Build history of the part. All positions in model axes, mm. A direction names the side the tool comes from. Round coordinates to 2 decimals unless told otherwise and drop trailing zeros. Write each loop counter-clockwise with the first axis right and the second up, starting at its lowest first coordinate (ties: lowest second). Pieces come first, ordered by that corner, then holes. Notation, with made-up numbers: (26, -35) -> (54, -35) arc R22 ccw to (54, -28) -> close; hole circle Ø2 at (86.5, 53). An arc over 180 degrees is marked (long way). Return JSON: item names as keys, results as strings.
from build123d import *

# Parameters (mm, degrees)
SKETCH_1_R          = 20
EXTRUDE_1_DEPTH     = 30
EXTRUDE_2_DEPTH     = 10
EXTRUDE_START       = -10
EXTRUDE_3_DEPTH     = 10
CUT_EXTRUDE_1_DEPTH = 30
SKETCH_6_W          = 120
SKETCH_6_H          = 10
CUT_EXTRUDE_2_DEPTH = 20
SKETCH_7_R          = 20
EXTRUDE_4_DEPTH     = 160


with BuildPart() as part:
    # 草图1 → 凸台-拉伸1 (new body)
    with BuildSketch(Plane.XY):
        with Locations((-197.711448945, 94.32879439)):
            Circle(SKETCH_1_R)
        with Locations((122.288551055, 94.32879439)):
            Circle(SKETCH_1_R)
        Polygon((-197.711448945, 114.32879439), (122.288551055, 114.32879439), (122.288551055, 74.32879439), (22.288551055, 74.32879439), (22.288551055, 14.32879439), (-97.711448945, 14.32879439), (-97.711448945, 74.32879439), (-197.711448945, 74.32879439), align=None)
    extrude(amount=EXTRUDE_1_DEPTH)

    # 草图3 → 凸台-拉伸2 (add)
    with BuildSketch(Plane(origin=(0, 0, 0), x_dir=(-1, 0, 0), z_dir=(0, 0, -1))):
        with BuildLine():
            ThreePointArc((97.711448945, 14.32879439), (37.711448945, 74.32879439), (-22.288551055, 14.32879439))
            Line((-22.288551055, 14.32879439), (97.711448945, 14.32879439))
        make_face()
        with BuildLine():
            Line((97.711448945, 14.32879439), (-22.288551055, 14.32879439))
            ThreePointArc((-22.288551055, 14.32879439), (37.711448945, -45.67120561), (97.711448945, 14.32879439))
        make_face()
    extrude(amount=-EXTRUDE_2_DEPTH)

    # 草图4 → 凸台-拉伸3 (add)
    with BuildSketch(Plane.XY.offset(30).offset(EXTRUDE_START)):
        with BuildLine():
            ThreePointArc((22.288551055, 14.32879439), (-37.711448945, 74.32879439), (-97.711448945, 14.32879439))
            Line((-97.711448945, 14.32879439), (22.288551055, 14.32879439))
        make_face()
        with BuildLine():
            Line((22.288551055, 14.32879439), (-97.711448945, 14.32879439))
            ThreePointArc((-97.711448945, 14.32879439), (-37.711448945, -45.67120561), (22.288551055, 14.32879439))
        make_face()
    extrude(amount=EXTRUDE_3_DEPTH)

    # 草图5 → 切除-拉伸1 (cut)
    with BuildSketch(Plane.XY.offset(30)):
        with BuildLine():
            ThreePointArc((-37.711448945, 6.32879439), (-46.130484457, 4.654144105), (-53.267798131, -0.114856424))
            Line((-53.267798131, -0.114856424), (-48.318050663, -5.064603892))
            ThreePointArc((-48.318050663, -5.064603892), (-43.45170043, -1.813012622), (-37.711448945, -0.67120561))
            Line((-37.711448945, -0.67120561), (-37.711448945, 6.32879439))
        make_face()
        with BuildLine():
            ThreePointArc((-22.155099759, -0.114856424), (-29.292413433, 4.654144105), (-37.711448945, 6.32879439))
            Line((-37.711448945, 6.32879439), (-37.711448945, -0.67120561))
            ThreePointArc((-37.711448945, -0.67120561), (-31.971197459, -1.813012622), (-27.104847227, -5.064603892))
            Line((-27.104847227, -5.064603892), (-22.155099759, -0.114856424))
        make_face()
        with BuildLine():
            ThreePointArc((-27.104847227, -5.064603892), (-31.971197459, -1.813012622), (-37.711448945, -0.67120561))
            Line((-37.711448945, -0.67120561), (-37.711448945, -15.67120561))
            Line((-37.711448945, -15.67120561), (-27.104847227, -5.064603892))
        make_face()
        with BuildLine():
            ThreePointArc((-37.711448945, -0.67120561), (-43.45170043, -1.813012622), (-48.318050663, -5.064603892))
            Line((-48.318050663, -5.064603892), (-37.711448945, -15.67120561))
            Line((-37.711448945, -15.67120561), (-37.711448945, -0.67120561))
        make_face()
        with BuildLine():
            Line((-37.711448945, -15.67120561), (-48.318050663, -5.064603892))
            ThreePointArc((-48.318050663, -5.064603892), (-43.45170043, -29.529398598), (-22.711448945, -15.67120561))
            ThreePointArc((-22.711448945, -15.67120561), (-23.853255957, -9.930954125), (-27.104847227, -5.064603892))
            Line((-27.104847227, -5.064603892), (-37.711448945, -15.67120561))
        make_face()
    extrude(amount=-CUT_EXTRUDE_1_DEPTH, mode=Mode.SUBTRACT)

    # 草图6 → 切除-拉伸2 (cut)
    with BuildSketch(Plane.XZ.offset(-14.32879439)):
        with Locations((-37.711448945, 15)):
            Rectangle(SKETCH_6_W, SKETCH_6_H)
    extrude(amount=-CUT_EXTRUDE_2_DEPTH, mode=Mode.SUBTRACT)

    # 草图7 → 凸台-拉伸4 (add)
    with BuildSketch(Plane.XY.offset(30)):
        with Locations(Location((-197.711448945, 94.32879439, 0), (0, 0, 90))):
            Circle(SKETCH_7_R)
        with Locations(Location((122.288551055, 94.32879439, 0), (0, 0, 90))):
            Circle(SKETCH_7_R)
    extrude(amount=EXTRUDE_4_DEPTH)


solid = part.part
Q1. Saw through at D-D on y = 65.5. List the corners of the cut face in (x, z).
Verdict:
{"outline": "(-97.71, 0) -> (22.29, 0) -> (22.29, 30) -> (-97.71, 30) -> close"}
Q2. Pin check, flat tips, straight feed: pin 1 Ø24 at (y, z) = (51.5, 22.5) entering from +X; pin 2 Ø10 at (y, z) = (-22.5, 32.5) entering from +X (3 decimals); pin 3 Ø24 at (x, y) = (-46.5, -16) entering from +Z. Stop position of each tip, or through.
Verdict:
{"pin 1": "stops at x = 22.29", "pin 2": "stops at x = 12.725", "pin 3": "stops at z = 30"}
Q3. Saw through at C-C on z = 41.5. List the corners of the cut face in (x, y).
Verdict:
{"outline": "circle Ø40 at (-197.71, 94.33); circle Ø40 at (122.29, 94.33)"}
Q4. Wall check: L1, parallel to Z at x = -79.5, y = -10; L2, parallel to Z at x = -154.5, y = 107; L3, parallel to Y at x = -88.5, z = 17.5. Give the ranges that are in metal, low to high.
Verdict:
{"L1": "z = 0 to 10, 20 to 30", "L2": "z = 0 to 30", "L3": "y = 34.33 to 114.33"}
Q5. Two-plate mould, pull along Z, no slides. Class faces 1 (the flat face through (-40, 53, 30)), 2 (the cylindrical face through (-36.392, -45.657, 4.93)), 3 (the flat face through (-39, 34.329, 15)), 4 (the flat face through (-35, 71, 0)): +Z half, -Z half, draft (parallel to the pull), parting line (faces both ways), or undercut.
Verdict:
{"face 1": "+Z half", "face 2": "draft", "face 3": "undercut", "face 4": "-Z half"}
Q6. Saw through at A-A on y = 25.5. List the corners of the cut face in (x, z).
Verdict:
{"outline": "(-97.71, 0) -> (22.29, 0) -> (22.29, 10) -> (-97.71, 10) -> close; (-97.71, 20) -> (22.29, 20) -> (22.29, 30) -> (-97.71, 30) -> close"}
Q7. Saw through at B-B on x = -13. List the corners of the cut face in (y, z), then the cut area to 3 significant figures.
Verdict:
{"outline": "(-40.35, 0) -> (114.33, 0) -> (114.33, 30) -> (-40.35, 30) -> (-40.35, 20) -> (34.33, 20) -> (34.33, 10) -> (-40.35, 10) -> close", "area": "3,890 mm²"}
Q8. 3-axis set-ups, long thin cutter, end or side, ignore diameter. For faces 5 (the flat face through (22.289, 45, 15)), 6 (the flat face through (-97.711, 44, 15)), 7 (the flat face through (-198, 94, 190)), 8 (the flat face through (-39, 12, 10)), 9 (the cylindrical face through (-217.54, 91.73, 93.67)): which of +Z, -Z, +X, -X, +Y, -Y reach the whole face in a straight line?
Verdict:
{"face 5": "+Z, -Z, +X, -Y", "face 6": "+Z, -Z, -X, -Y", "face 7": "+Z, +X, -X, +Y, -Y", "face 8": "+X, -X, -Y", "face 9": "+Z"}
